from build123d import *

# Parameters (mm, degrees)
F1_R      = 35
F2_DEPTH  = 35
F3_W      = 12
F3_H      = 3.6460709646
F3_H_2    = 3.3244666532
F5_R      = 4.0464813239
F5_R_2    = 2.5
F6_DEPTH  = 2
F7_COUNT  = 32
F8_R      = 1
F9_DEPTH  = 311.1
F10_R     = 6
F11_DEPTH = 1


with BuildPart() as f2:
    # F1 (on Top) → F2 (new body, symmetric)
    with BuildSketch(Plane.XY):
        Circle(F1_R)
    extrude(amount=F2_DEPTH, both=True)



with BuildPart() as f4:
    # F3 (on Front) → F4 (revolve)
    with BuildSketch(Plane.XZ):
        with Locations((-317, 10.1769645177)):
            Rectangle(F3_W, F3_H)
        with Locations((-317, -10.3377666734)):
            Rectangle(F3_W, F3_H_2)
        with BuildLine():
            ThreePointArc((-299, -11.9582607431), (-299.4995646481, -11.9895606449), (-300, -12))
            Line((-300, -12), (-299, -12))
            Line((-299, -12), (-299, -11.9582607431))
        make_face()
        with BuildLine():
            Line((-311, 12), (-311, 8.3539290354))
            Line((-311, 8.3539290354), (-311, -8.6755333468))
            Line((-311, -8.6755333468), (-311, -12))
            Line((-311, -12), (-300, -12))
            ThreePointArc((-300, -12), (-299.4995646481, -11.9895606449), (-299, -11.9582607431))
            ThreePointArc((-299, -11.9582607431), (-288, 0), (-299, 11.9582607431))
            ThreePointArc((-299, 11.9582607431), (-299.4995646481, 11.9895606449), (-300, 12))
            Line((-300, 12), (-311, 12))
        make_face()
    revolve(axis=Axis((0, 0, -12.4049474085), (0, 0, -1)))

    # F5 (on face) → F6 (join)
    with BuildSketch(Plane.XY.offset(12)):
        with Locations((0, -316.9144690037)):
            Circle(F5_R)
        with Locations((0, -316.9144690037)):
            Circle(F5_R_2, mode=Mode.SUBTRACT)
    extrude(amount=F6_DEPTH)

    # F7: F4 ×32 about axis
    f7_axis = Axis((0, 0, 35), (0, 0, 1))


with BuildPart() as f4_1:
    add(f4.part)
    for i in range(1, F7_COUNT):
        add(f4.part.rotate(f7_axis, i * 360 / F7_COUNT))


with BuildPart() as f2_1:
    add(f2.part)

    add(f4_1.part)  # F9 merges F4
    # F8 (on Front) → F9 (join)
    with BuildSketch(Plane.XZ):
        Circle(F8_R)
    extrude(amount=F9_DEPTH)

    # F10 (on face) → F11 (join)
    with BuildSketch(Plane.XZ.offset(311.1)):
        Circle(F10_R)
    extrude(amount=F11_DEPTH)


solid = f2_1.part
Verification items for the finished model (mm, model axes). A direction names the side the tool comes from. Give positions to 0.01 mm unless a question says otherwise; leave off trailing zeros. Order: outer loops, then holes, each group sorted by start corner. A loop starts at its lowest first (then second) coordinate and runs counter-clockwise, first axis right, second up. Notation, with made-up numbers: M 65,18.25 L 102,18.25 A16 ccw 102,38.25 Z; hole C 78.25,-17 d1. An arc over 180 degrees is marked long. Use one line per item in the form item = value. Start each with the question number.
Q1. Section check A-A (z = -22). Enter the section's corners in (x, y), then the cut area to 3 significant figures.
Q2. Access from +Z, -Z, +X, -X, +Y, -Y to the whole of each face (thin tool, end or side, straight path). Record for faces 4 (the flat face through (286, -94, 12)), 5 (the cylindrical face through (-308.084, 97.02, -10.314)), 6 (the flat face through (169, 265, 8.354)).
Q3. Mould release check, pull along X, two halves, no side actions. Record for faces 1 (the cylindrical face through (-28, -21, 0)), 2 (the flat face through (-94, -286, -12)), 3 (the cylindrical face through (-308.084, 97.02, 10.202)): +X half, -X half, draft (parallel to the pull), parting line (faces both ways), or undercut.
Q4. Go/stop test with flat-tipped pins: pin 1 Ø4 at (x, y) = (-176.07, 263.5) entering from -Z; pin 2 Ø3.5 at (x, z) = (-3, 0) entering from -Y; pin 3 Ø4 at (x, y) = (-309.5, 61) entering from +Z; pin 4 Ø4 at (y, z) = (93.5, 15) entering from -X. Record where each tip stops, or that it passes through.
Q5. Section check B-B (y = -97). Count the separate pieces of the cut face and the enclosed holes in it, then the cut area to 3 significant figures.
Q6. Scan lines: line 1 along Y through (x, z) = (0, 13); line 2 along Z through (x, y) = (-24, -297); line 3 along Y through (x, z) = (-76, 3.5). Record each from-to range of solid material in increasing order. Write a range as [from, to].
Evaluation:
q1.outline = C 0,0 d70
q1.area = 3,850 mm2
q2.face_4 = +Z
q2.face_5 = +Z, -Z
q2.face_6 = none
q3.face_1 = undercut
q3.face_2 = draft
q3.face_3 = parting line
q4.pin_1 = -12
q4.pin_2 = -312.1
q4.pin_3 = 14
q4.pin_4 = through
q5.separate_pieces = 3
q5.enclosed_holes = 0
q5.area = 1,210 mm2
q6.line_1 = [-320.96, -319.41], [-314.41, -312.87], [-35, 35], [312.87, 314.41], [319.41, 320.96]
q6.line_2 = [-11.83, 11.83]
q6.line_3 = [-301.57, -278.33], [278.33, 301.57]
